from build123d import *

# Parameters (mm, degrees)
SALIENTE_EXTRUIR1_DEPTH = 10
CROQUIS2_R              = 2.5
CORTAR_EXTRUIR1_DEPTH   = 21


with BuildPart() as part:
    # Croquis1 → Saliente-Extruir1 (new body)
    with BuildSketch(Plane.XY):
        with BuildLine():
            Line((-10, -15), (-10, -40))
            Line((-10, -40), (-3.5, -40))
            Line((-3.5, -40), (-3.5, -15))
            Line((-3.5, -15), (3.5, -15))
            Line((3.5, -15), (3.5, -40))
            Line((3.5, -40), (10, -40))
            Line((10, -40), (10, -15))
            Line((10, -15), (10, 15))
            Line((10, 15), (4.695324154, 15))
            ThreePointArc((4.695324154, 15), (0, 28.348412698), (-4.695324154, 15))
            Line((-4.695324154, 15), (-10, 15))
            Line((-10, 15), (-10, -15))
        make_face()
    extrude(amount=SALIENTE_EXTRUIR1_DEPTH)

    # Croquis2 → Cortar-Extruir1 (cut)
    with BuildSketch(Plane(origin=(10, 0, 0), x_dir=(0, 0, -1), z_dir=(1, 0, 0))):
        with Locations((-5, 12)):
            Circle(CROQUIS2_R)
    extrude(amount=-CORTAR_EXTRUIR1_DEPTH, mode=Mode.SUBTRACT)


solid = part.part
Work out the finished part from the listing and answer in its coordinate system (mm). A direction names the side the tool comes from. Round coordinates to 2 decimals unless told otherwise and drop trailing zeros. Write each loop counter-clockwise with the first axis right and the second up, starting at its lowest first coordinate (ties: lowest second). Pieces come first, ordered by that corner, then holes.
1) A cutting plane is placed at A-A (y = 12). Give the vertices of the cut face in (x, z), plus the area to 3 significant figures.
2) A cutting plane is placed at B-B (z = 5). Give the vertices of the cut face in (x, y).
3) A tool of negligible diameter and unlimited length cuts with its end or side. For faces 4 (the flat face through (-10, -12, 5)), 5 (the flat face through (0, -15, 5)), 6 (the flat face through (7, 15, 5)), 7 (the flat face through (-7, 15, 5)), 8 (the flat face through (0, -5, 10)), from which of +Z, -Z, +X, -X, +Y, -Y can it reach the whole face along a straight path? Write none if from no direction.
4) Straight lines are drawn through the part: line 1 (X direction, y = -29.5, z = 1.75); line 2 (Y direction, x = -0.25, z = 5.25); line 3 (Y direction, x = 6, z = 6.75). For each, find the intervals that lie inside material, in ascending order.
5) The mould has two halves that part along Z. Classify faces 1 (the flat face through (-7, -40, 5)), 2 (the flat face through (0, -5, 0)), 3 (the cylindrical face through (0.14, 9.78, 3.85)): pulls with the +Z half, pulls with the -Z half, needs draft (parallel to the pull), parting line crosses it, or undercut.
6) A cutting plane is placed at D-D (y = -20). Give the vertices of the cut face in (x, z).
7) Given pin 1 Ø1.5 at (x, z) = (-6, 4) entering from +Y; pin 2 Ø3.5 at (x, z) = (-1.5, 5) entering from -Y; pin 3 Ø6 at (x, z) = (7.5, 5.5) entering from +Y, each flat-ended and moving along its own axis, determine where each tip first touches the part or whether it passes through.
8) A cutting plane is placed at C-C (x = 0). Give the vertices of the cut face in (y, z).
Completed:
1. outline: (-10, 0) - (10, 0) - (10, 2.5) - (-10, 2.5) - close; (-10, 7.5) - (10, 7.5) - (10, 10) - (-10, 10) - close
1. area: 100 mm2
2. outline: (-10, -40) - (-3.5, -40) - (-3.5, -15) - (3.5, -15) - (3.5, -40) - (10, -40) - (10, 9.5) - (-10, 9.5) - close; (-10, 14.5) - (10, 14.5) - (10, 15) - (4.7, 15) arc R7.5 ccw (long way) to (-4.7, 15) - (-10, 15) - close
3. face 4: +Z, -Z, -X, +Y, -Y
3. face 5: +Z, -Z, -Y
3. face 6: +Z, -Z, +X
3. face 7: +Z, -Z, -X
3. face 8: +Z, +X, -X, +Y, -Y
4. line 1: x = -10 to -3.5, 3.5 to 10
4. line 2: y = -15 to 9.51, 14.49 to 28.34
4. line 3: y = -40 to 10.21, 13.79 to 15, 16.35 to 25.35
5. face 1: needs draft
5. face 2: pulls with the -Z half
5. face 3: undercut
6. outline: (-10, 0) - (-3.5, 0) - (-3.5, 10) - (-10, 10) - close; (3.5, 0) - (10, 0) - (10, 10) - (3.5, 10) - close
7. pin 1: stops at y = 26.2
7. pin 2: stops at y = -15
7. pin 3: stops at y = 26.85
8. outline: (-15, 0) - (28.35, 0) - (28.35, 10) - (-15, 10) - close; hole circle Ø5 at (12, 5)
